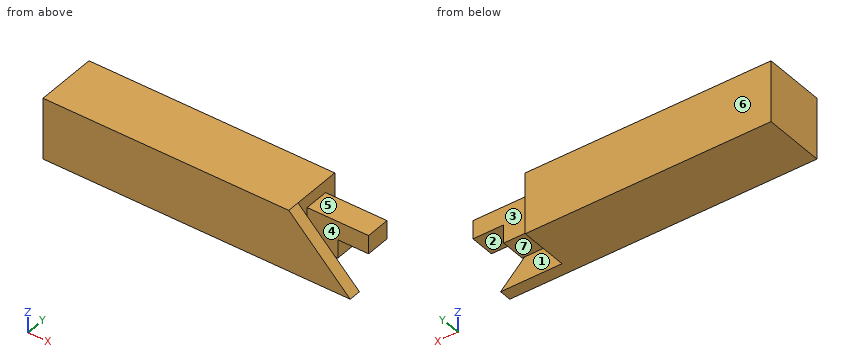
```python
from build123d import *

# Parameters (mm, degrees)
BOX004_W               = 25
BOX004_H               = 20
BOX004_DEPTH           = 20
BOX002_W               = 200
BOX002_H               = 50
BOX002_DEPTH           = 50
BOX003_W               = 50
BOX003_H               = 20
BOX003_DEPTH           = 30
BOX001_W               = 100
BOX001_H               = 10
BOX001_DEPTH           = 100
BOX001_PLACEMENT_ANGLE = 45
BOX_W                  = 50
BOX_H                  = 10
BOX_DEPTH              = 50


with BuildPart() as cube004:
    # Box004 → Box004 (new body)
    with BuildSketch(Plane(origin=(25, 20, 5), x_dir=(1, 0, 0), z_dir=(0, 0, 1))):
        with Locations((12.5, 10)):
            Rectangle(BOX004_W, BOX004_H)
    extrude(amount=BOX004_DEPTH)


with BuildPart() as cube002:
    # Box002 → Box002 (new body)
    with BuildSketch(Plane(origin=(0, 0, 50), x_dir=(-1, 0, 0), z_dir=(0, 0, -1))):
        with Locations((100, 25)):
            Rectangle(BOX002_W, BOX002_H)
    extrude(amount=BOX002_DEPTH)


with BuildPart() as cube003:
    # Box003 → Box003 (new body)
    with BuildSketch(Plane(origin=(0, 20, 10), x_dir=(1, 0, 0), z_dir=(0, 0, 1))):
        with Locations((25, 10)):
            Rectangle(BOX003_W, BOX003_H)
    extrude(amount=BOX003_DEPTH)


with BuildPart() as cube001:
    # Box001 → Box001 (new body)
    with BuildSketch(Plane.XY):
        with Locations((50, 5)):
            Rectangle(BOX001_W, BOX001_H)
    extrude(amount=BOX001_DEPTH)


with BuildPart() as cube001_1:
    # Box001 placement: moved
    add(cube001.part.moved(Location((0, 0, 50))).rotate(Axis((0, 0, 50), (0, 1, 0)), BOX001_PLACEMENT_ANGLE))


with BuildPart() as cut001:
    # Box → Box (new body)
    with BuildSketch(Plane.XY):
        with Locations((25, 5)):
            Rectangle(BOX_W, BOX_H)
    extrude(amount=BOX_DEPTH)

    # Cut: cut Cube001
    add(cube001_1.part, mode=Mode.SUBTRACT)

    # Fusion: union Cube002, Cube003
    add(cube002.part)
    add(cube003.part)

    # Cut001: cut Cube004
    add(cube004.part, mode=Mode.SUBTRACT)


solid = cut001.part
```
Geometry check sheet. Reference: the model listing, model coordinates, mm. Face numbers are marked on the shaded views. A direction names the side the tool comes from. Coordinates: 2 decimals unless noted, no trailing zeros. Loops run counter-clockwise (first coordinate to the right, second up) from the corner with the lowest first, then second, coordinate; pieces in that order, holes last. Notation, with made-up numbers: (58.5, 55.25) - (64.5, 55.25) arc R12 ccw to (64.5, 68.25) - close; hole circle Ø10 at (53.5, 12.25). An arc over 180 degrees is marked (long way). One line per item, written item: value. Start each with the question number.
(1) Mould release check, pull along Y, two halves, no side actions. Record for the marked faces 1, 2 and 3: released by +Y, released by -Y, zero draft, split by the parting line, or undercut.
(2) Cross-section at C-C on z = 45.5. Enter the section's corners in (x, y).
(3) Cross-section at B-B on y = 37. Enter the section's corners in (x, z), plus the area to 3 significant figures.
(4) Cross-section at A-A on z = 34. Enter the section's corners in (x, y), plus the area to 3 significant figures.
(5) Cross-section at D-D on y = 4.5. Enter the section's corners in (x, z).
(6) Material ranges on line 1 (Y direction, x = 4.5, z = 21.5); line 2 (X direction, y = 42.5, z = 33.5); line 3 (X direction, y = 20.5, z = 23), recorded low to high. Write a range as [from, to].
(7) Depth check by flat-ended pin: P1, Ø6, axis at x = 11.5, y = 34.5, coming from the -Z side; P2, Ø7.5, axis at y = 30, z = 20.5, coming from the +X side; P3, Ø9, axis at x = 19.5, z = 32, coming from the +Y side. Enter the tip coordinate at first touch or a pass-through.
(8) Tool access check on the marked faces 4, 5, 6 and 7. Record the directions out of +Z, -Z, +X, -X, +Y, -Y that give a thin tool (end or side, any length) a straight path to the whole face; none if there is none.
Results below:
1. face 1: undercut
1. face 2: zero draft
1. face 3: released by +Y
2. outline: (-200, 0) - (4.5, 0) - (4.5, 10) - (0, 10) - (0, 50) - (-200, 50) - close
3. outline: (-200, 0) - (0, 0) - (0, 10) - (25, 10) - (25, 25) - (50, 25) - (50, 40) - (0, 40) - (0, 50) - (-200, 50) - close
3. area: 11,100 mm2
4. outline: (-200, 0) - (16, 0) - (16, 10) - (0, 10) - (0, 20) - (50, 20) - (50, 40) - (0, 40) - (0, 50) - (-200, 50) - close
4. area: 11,200 mm2
5. outline: (-200, 0) - (50, 0) - (0, 50) - (-200, 50) - close
6. line 1: y = [0, 10], [20, 40]
6. line 2: x = [-200, 0]
6. line 3: x = [-200, 25]
7. P1: stops at z = 10
7. P2: stops at x = 25
7. P3: stops at y = 40
8. face 4: +Z, -Z, +X
8. face 5: +Z, +X, +Y
8. face 6: +Z, -Z, +X, -X, +Y
8. face 7: -Z, +X, +Y
